Read the model definition and answer for the solid it produces. Units are mm, in the model's axes. Coordinates: 2 decimals unless noted, no trailing zeros. Write each loop counter-clockwise with the first axis right and the second up, starting at its lowest first coordinate (ties: lowest second). Pieces come first, ordered by that corner, then holes. Notation, with made-up numbers: (26.5, 29.5) -> (54.5, 29.5) arc R33 cw to (54.5, 62.5) -> close; hole circle Ø11 at (40.5, 46). An arc over 180 degrees is marked (long way). One line per item, written item: value. Start each with the question number.
1. For a pull along X with two mould halves and no side action, classify faces 1 (the flat face through (-4, 5, 0)), 2 (the conical face through (20.797, 4.715, 8.348)), 3 (the cylindrical face through (16.98, -2.46, -0.78)) as pulls with the +X half, pulls with the -X half, needs draft (parallel to the pull), parting line crosses it, or undercut.
2. Given P1, Ø7, axis at x = -14.5, z = 0, coming from the +Y side; P2, Ø9, axis at x = 13.5, z = -1.5, coming from the +Y side; P3, Ø6, axis at x = 14.5, z = 0, coming from the -Y side, each flat-ended and moving along its own axis, determine where each tip first touches the part or whether it passes through.
3. Consider line 1 along X through (y, z) = (-2.25, 0); line 2 along X through (y, z) = (2.4, 0); line 3 along Z through (x, y) = (14.5, 2.2). Determine where each line is inside the solid, lowest interval first.
4. Find section D-D, the plane x = -14.5. Write down the section's boundary in (y, z).
5. Find section A-A, the plane x = 14.5. Write down the section's boundary in (y, z).
6. Find section C-C, the plane y = -0.75. Write down the section's boundary in (x, z).
7. Find section B-B, the plane z = 0. Write down the section's boundary in (x, y).
```python
from build123d import *

# Parameters (mm, degrees)
BOSS_EXTRUDE1_DEPTH = 22.5
SKETCH2_R           = 2.6
CUT_EXTRUDE1_DEPTH  = 11.5
SKETCH3_W           = 14
SKETCH3_H           = 20
CUT_EXTRUDE2_DEPTH  = 1.5
DRAFT1_ANGLE        = 45
FILLET1_R           = 4
SKETCH6_R           = 5.5
CUT_EXTRUDE3_DEPTH  = 5
CHAMFER2_SIZE       = 1


with BuildPart() as part:
    # Sketch1 → Boss-Extrude1 (new body, symmetric)
    with BuildSketch(Plane(origin=(0, 0, 0), x_dir=(0, 0, -1), z_dir=(1, 0, 0))):
        Polygon((-10, 5), (10, 5), (10, -5), (2.95, -5), (2.818767005, -6.5), (-2.818767005, -6.5), (-2.95, -5), (-10, -5), align=None)
    extrude(amount=BOSS_EXTRUDE1_DEPTH, both=True)

    # Sketch2 → Cut-Extrude1 (cut)
    with BuildSketch(Plane(origin=(0, 5, 0), x_dir=(1, 0, 0), z_dir=(0, 1, 0))):
        with Locations((-14.5, 0)):
            Circle(SKETCH2_R)
        with Locations((14.5, 0)):
            Circle(SKETCH2_R)
    extrude(amount=-CUT_EXTRUDE1_DEPTH, mode=Mode.SUBTRACT)

    # Sketch3 → Cut-Extrude2 (cut)
    with BuildSketch(Plane.XZ.offset(5)):
        with Locations((15.5, 0)):
            Rectangle(SKETCH3_W, SKETCH3_H)
        with Locations((-15.5, 0)):
            Rectangle(SKETCH3_W, SKETCH3_H)
    extrude(amount=CUT_EXTRUDE2_DEPTH, mode=Mode.SUBTRACT)

    # Draft1
    draft1_faces = [part.faces().sort_by_distance(p)[0] for p in [
        (8.5, -5.74431278, 0),
        (-8.5, -5.74431278, 0),
    ]]
    draft(draft1_faces, Plane(origin=(22.5, -6.5, -2.818767005), x_dir=(0, 0, -1), z_dir=(0, -1, 0)), DRAFT1_ANGLE)

    # Fillet1
    fillet1_edges = [part.edges().sort_by_distance(p)[0] for p in [
        (-22.5, 0, -10),
        (22.5, 0, 10),
        (22.5, 0, -10),
        (-22.5, 0, 10),
    ]]
    fillet(fillet1_edges, radius=FILLET1_R)

    # Sketch6 → Cut-Extrude3 (cut)
    with BuildSketch(Plane(origin=(0, 5, 0), x_dir=(1, 0, 0), z_dir=(0, 1, 0))):
        with Locations((14.5, 0)):
            Circle(SKETCH6_R)
    extrude(amount=-CUT_EXTRUDE3_DEPTH, mode=Mode.SUBTRACT)

    # Chamfer2
    chamfer2_edges = [part.edges().sort_by_distance(p)[0] for p in [
        (9, 5, 0),
        (22.5, 5, 0),
        (-22.5, 5, 0),
        (0, 5, 10),
        (0, 5, -10),
        (-21.328427125, 5, 8.828427125),
        (-21.328427125, 5, -8.828427125),
        (21.328427125, 5, 8.828427125),
        (21.328427125, 5, -8.828427125),
    ]]
    chamfer(chamfer2_edges, length=CHAMFER2_SIZE)


solid = part.part
```
Answer block:
1. face 1: needs draft
1. face 2: pulls with the +X half
1. face 3: undercut
2. P1: stops at y = 5
2. P2: stops at y = 4.8
2. P3: stops at y = -5
3. line 1: x = -22.5 to -17.1, -11.9 to 11.9, 17.1 to 22.5
3. line 2: x = -22.5 to -17.1, -11.9 to 9, 20 to 22.5
3. line 3: z = -10 to -5.5, 5.5 to 10
4. outline: (-5, -10) -> (4, -10) -> (5, -9) -> (5, -2.6) -> (-5, -2.6) -> close; (-5, 2.6) -> (5, 2.6) -> (5, 9) -> (4, 10) -> (-5, 10) -> close
5. outline: (-5, -10) -> (4, -10) -> (5, -9) -> (5, -6.5) -> (4, -5.5) -> (0, -5.5) -> (0, -2.6) -> (-5, -2.6) -> close; (-5, 2.6) -> (0, 2.6) -> (0, 5.5) -> (4, 5.5) -> (5, 6.5) -> (5, 9) -> (4, 10) -> (-5, 10) -> close
6. outline: (-22.5, -6) arc R4 ccw to (-18.5, -10) -> (18.5, -10) arc R4 ccw to (22.5, -6) -> (22.5, 6) arc R4 ccw to (18.5, 10) -> (-18.5, 10) arc R4 ccw to (-22.5, 6) -> close; hole circle Ø5.2 at (-14.5, 0); hole circle Ø5.2 at (14.5, 0)
7. outline: (-22.5, -5) -> (-17.1, -5) -> (-17.1, 5) -> (-21.5, 5) -> (-22.5, 4) -> close; (-11.9, -5) -> (-10, -5) -> (-8.5, -6.5) -> (8.5, -6.5) -> (10, -5) -> (11.9, -5) -> (11.9, 0) -> (9, 0) -> (9, 4) -> (8, 5) -> (-11.9, 5) -> close; (17.1, -5) -> (22.5, -5) -> (22.5, 4) -> (21.5, 5) -> (21, 5) -> (20, 4) -> (20, 0) -> (17.1, 0) -> close
